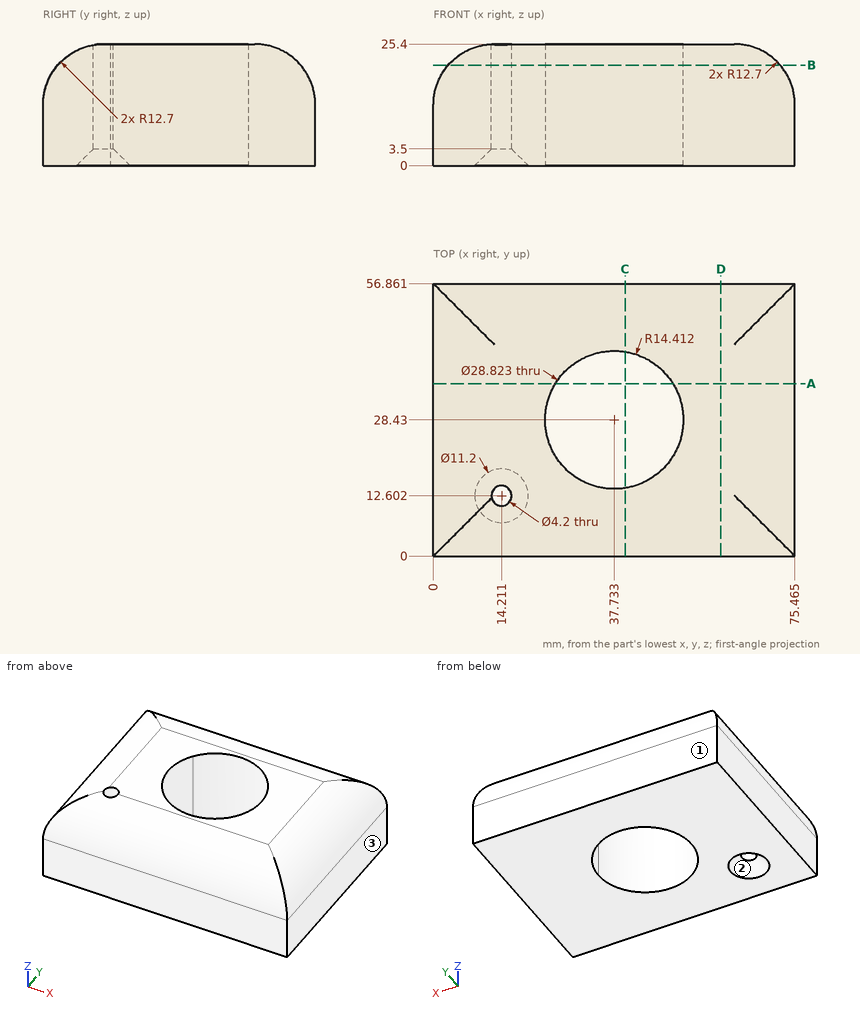
For this review, use the dimensioned drawing (mm, ordinates from the lowest corner) and the shaded views. Round coordinates to 2 decimals unless told otherwise and drop trailing zeros. Order: outer loops, then holes, each group sorted by start corner. A loop starts at its lowest first (then second) coordinate and runs counter-clockwise, first axis right, second up. Notation, with made-up numbers: M 43.25,48.5 L 100.25,48.5 A8 ccw 100.25,53.5 Z; hole C 1.25,65.25 d7. An arc over 180 degrees is marked long. Use a Markdown table: item, result. Add a question column.
Item 1: Mouldability with a two-part tool opening along X and no side actions: class the marked faces 1, 2 and 3 as released by +X, released by -X, zero draft, split by the parting line, or undercut.
Item 2: Add section B-B, the plane z = 21. Give the boundary of the cut face in (x, y) (1 decimal).
Item 3: Add section C-C, the plane x = 40. Give the boundary of the cut face in (y, z), then the cut area to 3 significant figures.
Item 4: Add section D-D, the plane x = 60. Give the boundary of the cut face in (y, z).
Item 5: To check wall thickness, follow line 1 along Y through (x, z) = (33, 18.5); line 2 along Y through (x, z) = (13, 19) (1 decimal); line 3 along X through (y, z) = (38, 18.25) (1 decimal). State the ranges of each line that lie inside material, in increasing order.
Item 6: Add section A-A, the plane y = 36. Give the boundary of the cut face in (x, z) (1 decimal).
Item 7: Insertion check: pin 1 (10 mm diameter, centred on y = 18.5, z = 19, fed in from +X); pin 2 (2 mm diameter, centred on x = 16.5, y = 12.5, fed in from -Z); pin 3 (5 mm diameter, centred on x = 50, z = 19.5, fed in from +Y); pin 4 (2 mm diameter, centred on x = 16.5, y = 26, fed in from -Z). Each pin has a flat end and moves straight along its axis. Give the tip position at first contact, or say it passes through.
Geometry results:
| question | item | result |
|---|---|---|
| 1 | face 1 | zero draft |
| 1 | face 2 | undercut |
| 1 | face 3 | released by +X |
| 2 | outline | M 3.1,3.1 L 72.4,3.1 L 72.4,53.8 L 3.1,53.8 Z; hole C 14.2,12.6 d4.2; hole C 37.7,28.4 d28.8 |
| 3 | outline | M 0,0 L 14.2,0 L 14.2,25.4 L 12.7,25.4 A12.7 ccw 0,12.7 Z; M 42.66,0 L 56.86,0 L 56.86,12.7 A12.7 ccw 44.16,25.4 L 42.66,25.4 Z |
| 3 | area | 652 mm² |
| 4 | outline | M 0,0 L 56.86,0 L 56.86,12.7 A12.7 ccw 44.16,25.4 L 12.7,25.4 A12.7 ccw 0,12.7 Z |
| 5 | line 1 | y = 1.4 to 14.82, 42.04 to 55.46 |
| 5 | line 2 | y = 1.7 to 10.9, 14.3 to 55.2 |
| 5 | line 3 | x = 1.3 to 27, 48.5 to 74.2 |
| 6 | outline | M 0,0 L 25.5,0 L 25.5,25.4 L 12.7,25.4 A12.7 ccw 0,12.7 Z; M 50,0 L 75.5,0 L 75.5,12.7 A12.7 ccw 62.8,25.4 L 50,25.4 Z |
| 7 | pin 1 | stops at x = 75.4 |
| 7 | pin 2 | stops at z = 2.31 |
| 7 | pin 3 | stops at y = 56.11 |
| 7 | pin 4 | stops at z = 0 |
